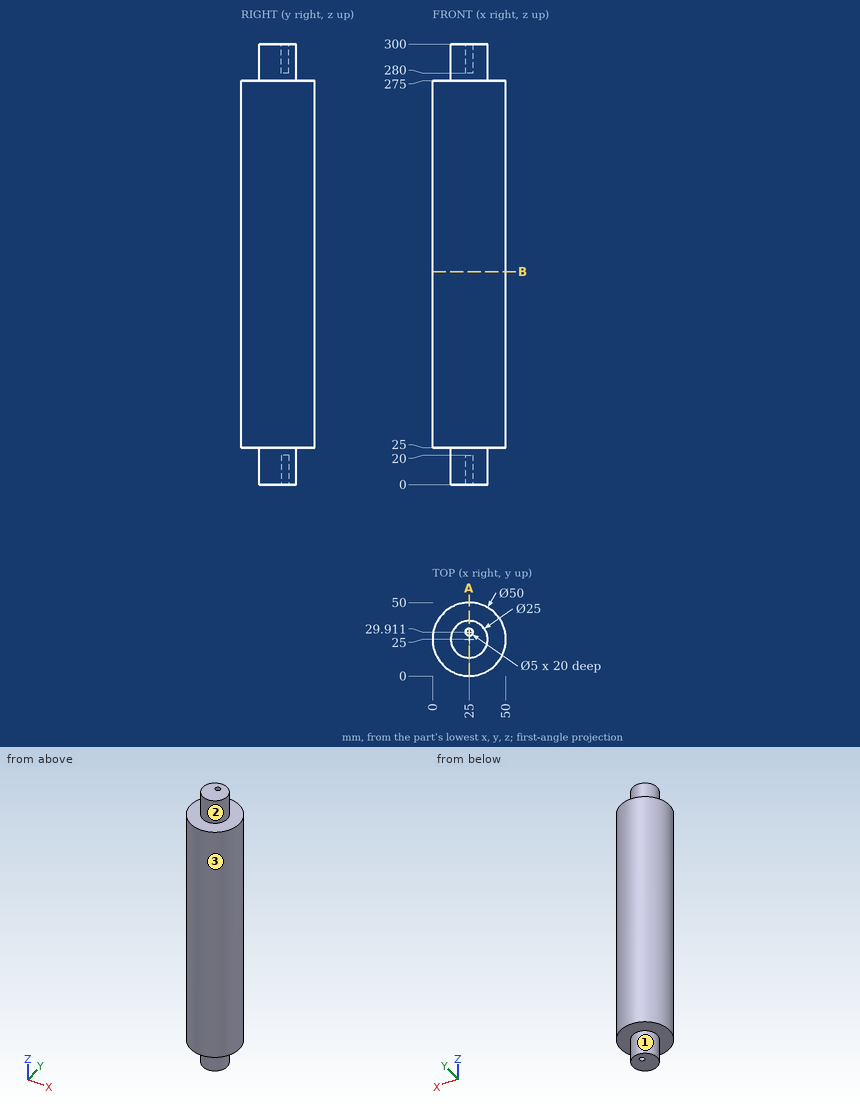
The drawing under review shows one solid part. Ordinate dimensions are in mm from its lowest x, y, z. A direction names the side the tool comes from. Give positions to 0.01 mm unless a question says otherwise; leave off trailing zeros. Loops run counter-clockwise (first coordinate to the right, second up) from the corner with the lowest first, then second, coordinate; pieces in that order, holes last. Notation, with made-up numbers: M 83,66 L 96,66 A29 cw 96,86 Z; hole C 73,74 d9. An arc over 180 degrees is marked long. One line per item, written item: value. Start each with the question number.
Q1. Add section A-A (x = 25). Give the boundary of the cut face in (y, z), and give its area (4 significant figures).
Q2. Add section B-B (z = 145). Give the boundary of the cut face in (x, y).
Q3. For L1, parallel to Y at x = 25, z = 5; L2, parallel to Z at x = 42, y = 24; L3, parallel to Y at x = 25, z = 275.5, list the stretches that pass through material, from the lowest coordinate up.
Q4. Machinability: for the marked faces 1, 2 and 3, which of the approach directions +Z, -Z, +X, -X, +Y, -Y give a long, thin tool a straight path to every point of the face, cutting with its end or side? Answer none if there is none.
Q5. Clearance check with flat-ended pins moving along their axes: pin 1 Ø2 at (y, z) = (38.5, 115.5) entering from -X; pin 2 Ø1.5 at (y, z) = (32.5, 173.5) entering from +X; pin 3 Ø10 at (y, z) = (34, 166) entering from -X. State where each tip first meets the part, or that it passes through.
Reply:
1. outline: M 0,25 L 12.5,25 L 12.5,0 L 27.41,0 L 27.41,20 L 32.41,20 L 32.41,0 L 37.5,0 L 37.5,25 L 50,25 L 50,275 L 37.5,275 L 37.5,300 L 32.41,300 L 32.41,280 L 27.41,280 L 27.41,300 L 12.5,300 L 12.5,275 L 0,275 Z
1. area: 13,550 mm²
2. outline: C 25,25 d50
3. L1: 12.5 to 27.41, 32.41 to 37.5
3. L2: 25 to 275
3. L3: 12.5 to 37.5
4. face 1: -Z
4. face 2: +Z
4. face 3: +Z, -Z
5. pin 1: x = 3.35
5. pin 2: x = 49.07
5. pin 3: x = 0.32
